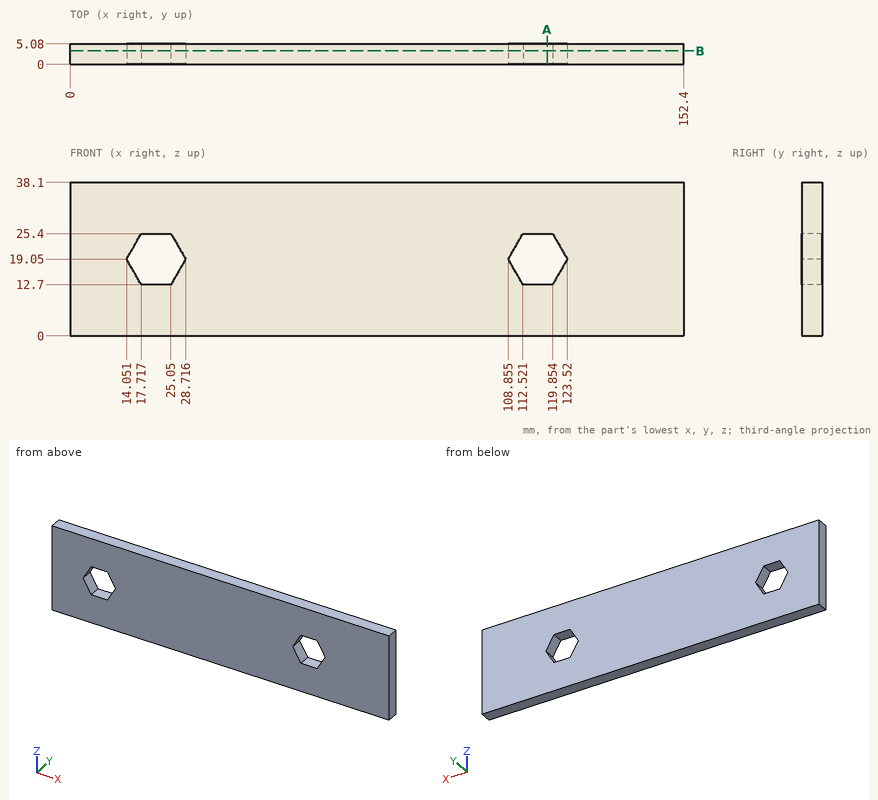
Study the drawing (mm; zero at the part's minimum x, y, z) and answer. Coordinates: 2 decimals unless noted, no trailing zeros. Write each loop counter-clockwise with the first axis right and the second up, starting at its lowest first coordinate (ties: lowest second). Pieces come first, ordered by that corner, then holes. Notation, with made-up numbers: (78.5, 0) - (128.5, 0) arc R13 cw to (128.5, 24) - close; hole circle Ø2 at (29.5, 83.25). An arc over 180 degrees is marked (long way). Return JSON: item names as keys, results as strings. Group by question number.
1. A cutting plane is placed at B-B, the plane y = 3.35. Give the number of separate pieces and of enclosed holes in the cut face, plus the area to 3 significant figures.
2. Straight lines are drawn through the part: L1, parallel to X at y = 2, z = 17 (1 decimal); L2, parallel to X at y = 4.8, z = 23 (1 decimal); L3, parallel to Z at x = 123, y = 1.8. For each, find the intervals that lie inside material, in ascending order.
3. A cutting plane is placed at A-A, the plane x = 118.5. Determine the outline of the cut face in (y, z), plus the area to 3 significant figures.
Ans:
{
 "1": {"separate pieces": "1", "enclosed holes": "2", "area": "5,530 mm²"},
 "2": {"L1": "0 to 15.2, 27.5 to 110, 122.3 to 152.4", "L2": "0 to 16.3, 26.4 to 111.1, 121.2 to 152.4", "L3": "0 to 18.15, 19.95 to 38.1"},
 "3": {"outline": "(0, 0) - (5.08, 0) - (5.08, 12.7) - (0, 12.7) - close; (0, 25.4) - (5.08, 25.4) - (5.08, 38.1) - (0, 38.1) - close", "area": "129 mm²"}
}
